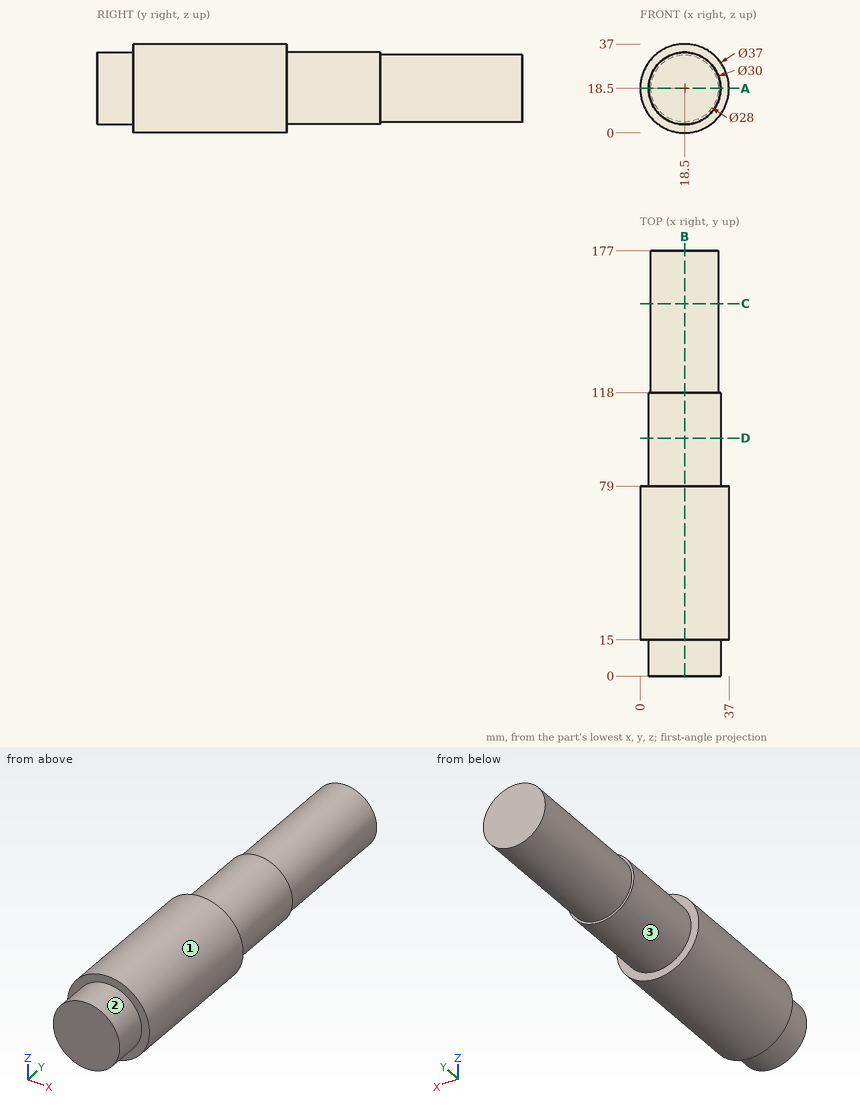
Input: dimensioned drawing with shaded views. Units: mm. Origin: part minimum x, y, z. A direction names the side the tool comes from. Round coordinates to 2 decimals unless told otherwise and drop trailing zeros. Loops run counter-clockwise (first coordinate to the right, second up) from the corner with the lowest first, then second, coordinate; pieces in that order, holes last.
1) Material intervals for line 1 (Z direction, x = 18, y = 97); line 2 (Y direction, x = 15.5, z = 3); line 3 (Z direction, x = 18.5, y = 24.5), sorted ascending.
Ans:
line 1: z = 3.51 to 33.49
line 2: y = 15 to 79
line 3: z = 0 to 37
2) Pin query (flat end, axial travel): pin 1 (2 mm diameter, centred on y = 55.5, z = 22.5, fed in from -X); pin 2 (12 mm diameter, centred on y = 22.5, z = 11.5, fed in from -X); pin 3 (1 mm diameter, centred on y = 69.5, z = 8.5, fed in from +X). Return the tip coordinate at first contact, or that it passes through.
Ans:
pin 1: stops at x = 0.24
pin 2: stops at x = 0.03
pin 3: stops at x = 34.37
3) Section query B-B on x = 18.5. Return the cut outline in (y, z), plus the area to 3 significant figures.
Ans:
outline: (0, 3.5) - (15, 3.5) - (15, 0) - (79, 0) - (79, 3.5) - (118, 3.5) - (118, 4.5) - (177, 4.5) - (177, 32.5) - (118, 32.5) - (118, 33.5) - (79, 33.5) - (79, 37) - (15, 37) - (15, 33.5) - (0, 33.5) - close
area: 5,640 mm2
4) Section query A-A on z = 18.5. Return the cut outline in (x, y).
Ans:
outline: (0, 15) - (3.5, 15) - (3.5, 0) - (33.5, 0) - (33.5, 15) - (37, 15) - (37, 79) - (33.5, 79) - (33.5, 118) - (32.5, 118) - (32.5, 177) - (4.5, 177) - (4.5, 118) - (3.5, 118) - (3.5, 79) - (0, 79) - close
5) Set-up query: the marked faces 1, 2 and 3. Return all of +Z, -Z, +X, -X, +Y, -Y with unobstructed straight access to the full face (end or side cutting, diameter ignored); none if empty.
Ans:
face 1: +Y, -Y
face 2: -Y
face 3: +Y
6) Section query D-D on y = 99. Return the cut outline in (x, z).
Ans:
outline: circle Ø30 at (18.5, 18.5)
7) Section query C-C on y = 155. Return the cut outline in (x, z).
Ans:
outline: circle Ø28 at (18.5, 18.5)
